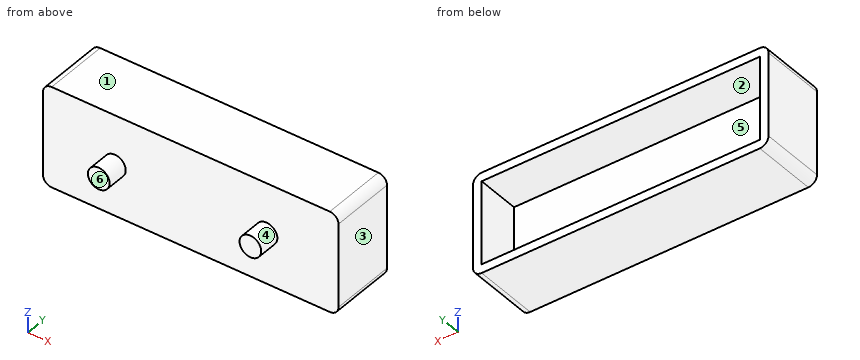
```python
from build123d import *

# Parameters (mm, degrees)
SKETCH1_W           = 68.2
SKETCH1_H           = 23.2
SKETCH1_W_2         = 64.2
SKETCH1_H_2         = 19.2
BOSS_EXTRUDE1_DEPTH = 10
SKETCH1_2_W         = 68.2
SKETCH1_2_H         = 23.2
SKETCH1_2_W_2       = 64.2
SKETCH1_2_H_2       = 19.2
BOSS_EXTRUDE2_DEPTH = 5
SKETCH2_R           = 2.5
BOSS_EXTRUDE3_DEPTH = 5
FILLET1_R           = 2


with BuildPart() as part:
    # Sketch1 → Boss-Extrude1 (new body)
    with BuildSketch(Plane(origin=(0, 0, 0), x_dir=(1, 0, 0), z_dir=(0, 1, 0))):
        with Locations((32.1, 9.6)):
            Rectangle(SKETCH1_W, SKETCH1_H)
        with Locations((32.1, 9.6)):
            Rectangle(SKETCH1_W_2, SKETCH1_H_2, mode=Mode.SUBTRACT)
    extrude(amount=BOSS_EXTRUDE1_DEPTH)

    # Sketch1_2 → Boss-Extrude2 (add)
    # profile 1 of 2: a face of its own
    with BuildSketch(Plane(origin=(0, 0, 0), x_dir=(1, 0, 0), z_dir=(0, 1, 0))):
        with Locations((32.1, 9.6)):
            Rectangle(SKETCH1_2_W, SKETCH1_2_H)
        with Locations((32.1, 9.6)):
            Rectangle(SKETCH1_2_W_2, SKETCH1_2_H_2, mode=Mode.SUBTRACT)
    # profile 2 of 2: a face of its own
    with BuildSketch(Plane(origin=(0, 0, 0), x_dir=(1, 0, 0), z_dir=(0, 1, 0))):
        with Locations((32.1, 9.6)):
            Rectangle(SKETCH1_2_W_2, SKETCH1_2_H_2)
    extrude(amount=-BOSS_EXTRUDE2_DEPTH)

    # Sketch2 → Boss-Extrude3 (add)
    with BuildSketch(Plane.XZ.offset(5)):
        with Locations(Location((14.6, -9.6, 0), (0, 0, 90))):
            Circle(SKETCH2_R)
        with Locations(Location((49.6, -9.6, 0), (0, 0, 90))):
            Circle(SKETCH2_R)
    extrude(amount=BOSS_EXTRUDE3_DEPTH)

    # Fillet1
    fillet1_edges = [part.edges().sort_by_distance(p)[0] for p in [
        (-2, 2.5, 2),
        (-2, 2.5, -21.2),
        (66.2, 2.5, -21.2),
        (66.2, 2.5, 2),
    ]]
    fillet(fillet1_edges, radius=FILLET1_R)


solid = part.part
```
Part model, mm, in its own coordinate system. Face numbers are marked on the shaded views. A direction names the side the tool comes from. Round coordinates to 2 decimals unless told otherwise and drop trailing zeros. Order: outer loops, then holes, each group sorted by start corner. A loop starts at its lowest first (then second) coordinate and runs counter-clockwise, first axis right, second up. Notation, with made-up numbers: M 44,1 L 86,1 A15 cw 86,11 Z; hole C 13.25,-3 d9. An arc over 180 degrees is marked long. Answer in a Markdown table with one row per item. Add a question column.
Q1. Cut at D-D on x = 14.6. Give the cut face in (y, z), and give its area (3 significant figures).
Q2. Cut at A-A on y = 5.5. Give the cut face in (x, z).
Q3. Pin check, flat tips, straight feed: pin 1 (6 mm diameter, centred on x = 34, z = -7, fed in from +Y); pin 2 (12 mm diameter, centred on x = 59.5, z = -8, fed in from -Y); pin 3 (12 mm diameter, centred on x = 54.5, z = -15, fed in from -Y). Stop position of each tip, or through.
Q4. Mould opens along X. For the marked faces 1, 2 and 3 say: +X half, -X half, draft (parallel to the pull), parting line (faces both ways), or undercut.
Q5. 3-axis set-ups, long thin cutter, end or side, ignore diameter. For the marked faces 4, 5 and 6: which of +Z, -Z, +X, -X, +Y, -Y reach the whole face in a straight line?
Q6. Cut at C-C on z = -3. Give the cut face in (x, y), and give its area (3 significant figures).
Q7. Wall check: L1, parallel to Z at x = 5, y = 1.5; L2, parallel to X at y = 6.75, z = -14.5; L3, parallel to Y at x = 62, z = -6. Give the ranges that are in metal, low to high. Write a range as from..to.
Q8. Cut at B-B on x = 22. Give the cut face in (y, z), and give its area (3 significant figures).
Established:
| question | item | result |
|---|---|---|
| 1 | outline | M -10,-12.1 L -5,-12.1 L -5,-21.2 L 10,-21.2 L 10,-19.2 L 0,-19.2 L 0,0 L 10,0 L 10,2 L -5,2 L -5,-7.1 L -10,-7.1 Z |
| 1 | area | 181 mm2 |
| 2 | outline | M -2,-19.2 A2 ccw 0,-21.2 L 64.2,-21.2 A2 ccw 66.2,-19.2 L 66.2,0 A2 ccw 64.2,2 L 0,2 A2 ccw -2,0 Z; hole M 0,-19.2 L 64.2,-19.2 L 64.2,0 L 0,0 Z |
| 3 | pin 1 | stops at y = 0 |
| 3 | pin 2 | stops at y = -5 |
| 3 | pin 3 | stops at y = -10 |
| 4 | face 1 | draft |
| 4 | face 2 | undercut |
| 4 | face 3 | +X half |
| 5 | face 4 | -Y |
| 5 | face 5 | +Y |
| 5 | face 6 | +Z, -Z, +X, -X, -Y |
| 6 | outline | M -2,-5 L 66.2,-5 L 66.2,10 L 64.2,10 L 64.2,0 L 0,0 L 0,10 L -2,10 Z |
| 6 | area | 381 mm2 |
| 7 | L1 | z = -21.2..-19.2, 0..2 |
| 7 | L2 | x = -2..0, 64.2..66.2 |
| 7 | L3 | y = -5..0 |
| 8 | outline | M -5,-21.2 L 10,-21.2 L 10,-19.2 L 0,-19.2 L 0,0 L 10,0 L 10,2 L -5,2 Z |
| 8 | area | 156 mm2 |
